Autodesk Inventor part; units mm, degrees
ref_plane "YZ Plane" through (0, 0, 0) normal (1, 0, 0) x (0, 1, 0)
ref_plane "XZ Plane" through (0, 0, 0) normal (0, 1, 0) x (-1, 0, 0)
ref_plane "XY Plane" through (0, 0, 0) normal (0, 0, 1) x (1, 0, 0)
sketch "Sketch1" plane through (0, 0, 0) normal (1, 0, 0) x (0, 1, 0)
  line L0 (0, 0) -> (0, -101.6)
  line L1 (0, -101.6) -> (-25.4, -101.6)
  line L2 (-25.4, -101.6) -> (-88.9, -50.8)
  line L3 (-88.9, -50.8) -> (-88.9, 0)
  circle A0 centre (-50.8, -12.7) radius 3.175
  circle A1 centre (-12.7, -50.8) radius 3.175
  circle A2 centre (-12.7, -88.9) radius 3.175
  line L4 (-12.7, -25.4) -> (-12.7, -101.6) construction
  line L5 (0, -12.7) -> (-88.9, -12.7) construction
  circle A3 centre (-76.2, -38.1) radius 3.175
  circle A4 centre (-25.4, -25.4) radius 14.2875
  line L6 (0, 0) -> (-88.9, 0)
  dimension "d0" = 50.8
  dimension "d1" = 25.4
  dimension "d2" = 88.9
  dimension "d3" = 101.6
  dimension "d5" = 38.1
  dimension "d6" = 12.7
  dimension "d10" = 12.7
  dimension "d11" = 12.7
  dimension "d13" = 28.575
  dimension "d15" = 6.35
  dimension "d24" = 90
  dimension "d25" = 12.7
  dimension "d26" = 25.4
  dimension "d27" = 76.2
  dimension "d29" = 63.5
  dimension "d30" = 6.35
  dimension "d31" = 50.8
  dimension "d32" = 38.1
extrude "Extrusion1" add sketch "Sketch1" along normal blind 3.175
sketch "Sketch2" plane through (3.175, 0, 0) normal (1, 0, 0) x (0, 0, -1)
  line L0 (50.8, -39.1889) -> (50.8, -28.575)
  line L1 (53.975, -25.4) -> (62.4661, -25.4)
  line L2 (64.9454, -30.5584) -> (56.4543, -41.1723)
  line L3 (101.6, 0) -> (0, 0)
  line L4 (0, 0) -> (0, -101.6)
  line L5 (50.8, -88.9) -> (101.6, -25.4)
  arc A0 (50.8, -39.1889) -> (56.4543, -41.1723) centre (53.975, -39.1889) ccw
  arc A1 (53.975, -25.4) -> (50.8, -28.575) centre (53.975, -28.575) ccw
  arc A2 (64.9454, -30.5584) -> (62.4661, -25.4) centre (62.4661, -28.575) ccw
  line L6 (0, 0) -> (0, -88.9)
  dimension "d18" = 25.4
  dimension "d19" = 25.4
  dimension "d21" = 3.175
  dimension "d28" = 50.8
extrude "Extrusion2" cut sketch "Sketch2" against normal blind 3.175
properties part number "15102898-16-P-0205_CPY" material "Aluminum 6061"
Input: part model. Units: mm. Frame: model coordinates. A direction names the side the tool comes from. Round coordinates to 2 decimals unless told otherwise and drop trailing zeros. Loops run counter-clockwise (first coordinate to the right, second up) from the corner with the lowest first, then second, coordinate; pieces in that order, holes last. Notation, with made-up numbers: (-22, 32.25) -> (32, 32.25) arc R12 ccw to (32, 37.25) -> close; hole circle Ø1 at (9, 84). An arc over 180 degrees is marked (long way). Answer as a JSON object with one key per item and string values. Group by question number.
1) Ray query, L1, parallel to Z at x = 0.85, y = -31; L2, parallel to Y at x = 1.05, z = -37; L3, parallel to Y at x = 0.75, z = -38.5. Return the intervals inside material, ascending.
2) Section query A-A on z = -88.9. Output: boundary loops of the cut face in (x, y) (3 decimals), plus the area to 3 significant figures.
3) Reachability of faces 4 (the cylindrical face through (1.61, -26.31, -51.75)), 5 (the flat face through (2, -44, 0)) from +Z, -Z, +X, -X, +Y, -Y: full face, straight path, thin tool, end or side. Return the list, or none.
4) Pin query (flat end, axial travel): pin 1 (8.5 mm diameter, centred on y = -50.8, z = -12.7, fed in from -X); pin 2 (2 mm diameter, centred on y = -36.5, z = -31.5, fed in from -X); pin 3 (1.5 mm diameter, centred on x = 1, y = -50, fed in from -Z); pin 4 (1.6 mm diameter, centred on x = 1, z = -59.5, fed in from -Y) (3 decimals). Return the tip coordinate at first contact, or that it passes through.
5) Section query D-D on z = -12.7. Output: boundary loops of the cut face in (x, y) (3 decimals).
6) Section query C-C on y = -17.5. Output: boundary loops of the cut face in (x, z) (3 decimals), plus the area to 3 significant figures.
7) Section query B-B on x = 1.45. State how many separate pieces and enclosed holes the cut face has, plus the area to 3 significant figures.
8) Draft query along Y for faces 1 (the flat face through (1.565, -56.705, -76.556)), 2 (the flat face through (3.175, -45, -50)), 3 (the cylindrical face through (1.57, -53.97, -12.84)). Return one class per face: +Y half, -Y half, draft (parallel to the pull), parting line (faces both ways), or undercut.
Reply:
{
 "1": {"L1": "z = -97.12 to -64.59, -50.8 to -38.54, -12.26 to 0", "L2": "y = -88.9 to -79.18, -73.22 to -33.74, -17.06 to 0", "L3": "y = -88.9 to -79.35, -73.05 to -31.1, -19.7 to 0"},
 "2": {"outline": "(0, -41.275) -> (3.175, -41.275) -> (3.175, -15.875) -> (0, -15.875) -> close; (0, -9.525) -> (3.175, -9.525) -> (3.175, 0) -> (0, 0) -> close", "area": "111 mm2"},
 "3": {"face 4": "+X, -X", "face 5": "+Z, +X, -X, +Y, -Y"},
 "4": {"pin 1": "stops at x = 0", "pin 2": "passes through", "pin 3": "stops at z = -82.52", "pin 4": "stops at y = -79.025"},
 "5": {"outline": "(0, -88.9) -> (3.175, -88.9) -> (3.175, -53.975) -> (0, -53.975) -> close; (0, -47.625) -> (3.175, -47.625) -> (3.175, -31.945) -> (0, -31.945) -> close; (0, -18.855) -> (3.175, -18.855) -> (3.175, 0) -> (0, 0) -> close"},
 "6": {"outline": "(0, -101.6) -> (3.175, -101.6) -> (3.175, -37.305) -> (0, -37.305) -> close; (0, -13.495) -> (3.175, -13.495) -> (3.175, 0) -> (0, 0) -> close", "area": "247 mm2"},
 "7": {"separate pieces": "1", "enclosed holes": "6", "area": "6,470 mm2"},
 "8": {"face 1": "-Y half", "face 2": "draft", "face 3": "undercut"}
}
